```python
from build123d import *

# Parameters (mm, degrees)
BOSS_EXTRUDE1_DEPTH    = 42
SKETCH4_W              = 14.859
SKETCH4_H              = 30
CUT_EXTRUDE2_DEPTH     = 6.35
SKETCH6_R              = 2.35
CUT_EXTRUDE3_DEPTH     = 6.35
CUT_EXTRUDE4_REACH     = 49.295
SKETCH7_R              = 1.625
CONVERT_SOLID1_DEPTH   = 6.254
CONVERT_SOLID1_START   = 35.746
CONVERT_SOLID1_2_DEPTH = 6.254
CONVERT_SOLID1_START_2 = 5.746
CONVERT_SOLID1_3_DEPTH = 0.508
CONVERT_SOLID1_4_DEPTH = 0.508
CONVERT_SOLID1_5_DEPTH = 5.746
CONVERT_SOLID1_START_3 = 36.254
CONVERT_SOLID1_6_DEPTH = 5.746


# Read off the part's stored shape, not the designer's step: Convert-Solid1
with BuildPart() as part:
    # Sketch1 → Boss-Extrude1 (new body)
    with BuildSketch(Plane(origin=(0, 0, 0), x_dir=(1, 0, 0), z_dir=(0, 1, 0))):
        Polygon((0, 0), (15.875, 0), (15.875, 1.016), (1.016, 1.016), (1.016, 15.875), (0, 15.875), align=None)
    extrude(amount=BOSS_EXTRUDE1_DEPTH)

    # Sketch4 → Cut-Extrude2 (cut)
    with BuildSketch(Plane(origin=(1.016, 0, 0), x_dir=(0, 0, -1), z_dir=(1, 0, 0))):
        with Locations((8.4455, 21)):
            Rectangle(SKETCH4_W, SKETCH4_H)
    extrude(amount=-CUT_EXTRUDE2_DEPTH, mode=Mode.SUBTRACT)

    # Sketch6 → Cut-Extrude3 (cut)
    with BuildSketch(Plane(origin=(1.016, 0, 0), x_dir=(0, 0, -1), z_dir=(1, 0, 0))):
        with Locations((7.666, 3.35)):
            Circle(SKETCH6_R)
        with Locations((7.666, 38.65)):
            Circle(SKETCH6_R)
    extrude(amount=-CUT_EXTRUDE3_DEPTH, mode=Mode.SUBTRACT)

    # Sketch7 → Cut-Extrude4 (cut, up to next)
    with BuildSketch(Plane(origin=(0, 0, -1.016), x_dir=(-1, 0, 0), z_dir=(0, 0, -1)), mode=Mode.PRIVATE) as cut_extrude4_sk1:
        with Locations((-8.4455, 39)):
            Circle(SKETCH7_R)
    cut_extrude4_tool1 = extrude(cut_extrude4_sk1.sketch, amount=-CUT_EXTRUDE4_REACH, mode=Mode.PRIVATE) & part.part
    # Sketch7 → Cut-Extrude4 (cut, up to next)
    with BuildSketch(Plane(origin=(0, 0, -1.016), x_dir=(-1, 0, 0), z_dir=(0, 0, -1)), mode=Mode.PRIVATE) as cut_extrude4_sk2:
        with Locations((-8.4455, 3)):
            Circle(SKETCH7_R)
    cut_extrude4_tool2 = extrude(cut_extrude4_sk2.sketch, amount=-CUT_EXTRUDE4_REACH, mode=Mode.PRIVATE) & part.part
    add(cut_extrude4_tool1.solids().sort_by_distance((8.4455, 39, -1.016))[0], mode=Mode.SUBTRACT)
    add(cut_extrude4_tool2.solids().sort_by_distance((8.4455, 3, -1.016))[0], mode=Mode.SUBTRACT)

    # Convert-Solid1 outline → Convert-Solid1 (cut)
    with BuildSketch(Plane(origin=(0, 0, 0), x_dir=(1, 0, 0), z_dir=(0, 1, 0))):
        with BuildLine():
            Line((0, 0), (2.016, 0))
            ThreePointArc((2.016, 0), (0.590472729, 0.590472729), (0, 2.016))
            Line((0, 2.016), (0, 0))
        make_face()
    extrude(amount=CONVERT_SOLID1_DEPTH, mode=Mode.SUBTRACT)

    # Convert-Solid1 2 outline → Convert-Solid1 2 (cut)
    with BuildSketch(Plane(origin=(0, 0, 0), x_dir=(1, 0, 0), z_dir=(0, 1, 0)).offset(CONVERT_SOLID1_START)):
        with BuildLine():
            Line((0, 0), (2.016, 0))
            ThreePointArc((2.016, 0), (0.590472729, 0.590472729), (0, 2.016))
            Line((0, 2.016), (0, 0))
        make_face()
    extrude(amount=CONVERT_SOLID1_2_DEPTH, mode=Mode.SUBTRACT)

    # Convert-Solid1 3 outline → Convert-Solid1 3 (cut)
    with BuildSketch(Plane(origin=(0, 0, 0), x_dir=(1, 0, 0), z_dir=(0, 1, 0)).offset(CONVERT_SOLID1_START_2)):
        with BuildLine():
            Line((2.016, 0), (3.54, 0))
            Line((3.54, 0), (3.54, 1.016))
            Line((3.54, 1.016), (1.016, 1.016))
            Line((1.016, 1.016), (1.016, 3.54))
            Line((1.016, 3.54), (0, 3.54))
            Line((0, 3.54), (0, 2.016))
            ThreePointArc((0, 2.016), (0.590472729, 0.590472729), (2.016, 0))
        make_face()
    extrude(amount=CONVERT_SOLID1_3_DEPTH, mode=Mode.SUBTRACT)

    # Convert-Solid1 4 outline → Convert-Solid1 4 (cut)
    with BuildSketch(Plane(origin=(0, 0, 0), x_dir=(1, 0, 0), z_dir=(0, 1, 0)).offset(CONVERT_SOLID1_START)):
        with BuildLine():
            Line((2.016, 0), (3.54, 0))
            Line((3.54, 0), (3.54, 1.016))
            Line((3.54, 1.016), (1.016, 1.016))
            Line((1.016, 1.016), (1.016, 3.54))
            Line((1.016, 3.54), (0, 3.54))
            Line((0, 3.54), (0, 2.016))
            ThreePointArc((0, 2.016), (0.590472729, 0.590472729), (2.016, 0))
        make_face()
    extrude(amount=CONVERT_SOLID1_4_DEPTH, mode=Mode.SUBTRACT)

    # Convert-Solid1 5 outline → Convert-Solid1 5 (add)
    with BuildSketch(Plane(origin=(0, 0, 0), x_dir=(1, 0, 0), z_dir=(0, 1, 0))):
        with BuildLine():
            Line((1.016, 1.016), (2.016, 1.016))
            ThreePointArc((2.016, 1.016), (1.308893219, 1.308893219), (1.016, 2.016))
            Line((1.016, 2.016), (1.016, 1.016))
        make_face()
    extrude(amount=CONVERT_SOLID1_5_DEPTH)

    # Convert-Solid1 6 outline → Convert-Solid1 6 (add)
    with BuildSketch(Plane(origin=(0, 0, 0), x_dir=(1, 0, 0), z_dir=(0, 1, 0)).offset(CONVERT_SOLID1_START_3)):
        with BuildLine():
            Line((1.016, 1.016), (2.016, 1.016))
            ThreePointArc((2.016, 1.016), (1.308893219, 1.308893219), (1.016, 2.016))
            Line((1.016, 2.016), (1.016, 1.016))
        make_face()
    extrude(amount=CONVERT_SOLID1_6_DEPTH)


solid = part.part
```
Check sheet for the modelled part. Datum: model origin and axes. Units: mm. A direction names the side the tool comes from. Coordinates: 2 decimals unless noted, no trailing zeros. Write each loop counter-clockwise with the first axis right and the second up, starting at its lowest first coordinate (ties: lowest second). Pieces come first, ordered by that corner, then holes. Notation, with made-up numbers: (35, 85) -> (73, 85) arc R15 ccw to (73, 106) -> close; hole circle Ø11 at (-3, 52). An arc over 180 degrees is marked (long way). Use a Markdown table: item, result.
1. Tool access check on faces 1 (the flat face through (0.5, 36, -9.6)), 2 (the flat face through (1, 36.254, -1)), 3 (the flat face through (1.016, 39, -10.4)), 4 (the cylindrical face through (0.61, 39.09, -0.57)). Record the directions out of +Z, -Z, +X, -X, +Y, -Y that give a thin tool (end or side, any length) a straight path to the whole face; none if there is none.
Reported:
| item | result |
|---|---|
| face 1 | +Z, -Z, +X, -X |
| face 2 | +Z, -X |
| face 3 | -Z, +X, +Y, -Y |
| face 4 | +Z, -X, +Y |
2. Sectioned sample at B-B (z = -12.5). Enter the section's corners in (x, y).
Reported:
| item | result |
|---|---|
| outline | (0, 0) -> (1.02, 0) -> (1.02, 6) -> (0, 6) -> close; (0, 36) -> (1.02, 36) -> (1.02, 42) -> (0, 42) -> close |
3. Sectioned sample at D-D (y = 25). Enter the section's corners in (x, z) (3 decimals).
Reported:
| item | result |
|---|---|
| outline | (0, -1.016) -> (15.875, -1.016) -> (15.875, 0) -> (0, 0) -> close |
4. Sectioned sample at C-C (z = -8.25). Enter the section's corners in (x, y).
Reported:
| item | result |
|---|---|
| outline | (0, 0) -> (1.02, 0) -> (1.02, 1.07) -> (0, 1.07) -> close; (0, 5.63) -> (1.02, 5.63) -> (1.02, 6) -> (0, 6) -> close; (0, 36) -> (1.02, 36) -> (1.02, 36.37) -> (0, 36.37) -> close; (0, 40.93) -> (1.02, 40.93) -> (1.02, 42) -> (0, 42) -> close |
5. Release check for a two-part mould opening along Y. For faces 5 (the cylindrical face through (0.61, 2.83, -0.57)), 6 (the flat face through (0.8, 42, -4.4)), 7 (the flat face through (0.5, 6, -9.6)) record: pulls with the +Y half, pulls with the -Y half, needs draft (parallel to the pull), parting line crosses it, or undercut.
Reported:
| item | result |
|---|---|
| face 5 | needs draft |
| face 6 | pulls with the +Y half |
| face 7 | undercut |
6. Go/stop test with flat-tipped pins: pin 1 Ø1 at (x, y) = (7.5, 21.5) entering from +Z; pin 2 Ø3 at (x, y) = (8.45, 3) entering from +Z; pin 3 Ø6.5 at (y, z) = (40.5, -10.5) entering from +X. Record where each tip stops, or that it passes through.
Reported:
| item | result |
|---|---|
| pin 1 | stops at z = 0 |
| pin 2 | passes through |
| pin 3 | stops at x = 1.02 |
7. Scan lines: line 1 along Z through (x, y) = (14, 29.5); line 2 along X through (y, z) = (37, -14.25). Record each from-to range of solid material in increasing order.
Reported:
| item | result |
|---|---|
| line 1 | z = -1.02 to 0 |
| line 2 | x = 0 to 1.02 |
8. Sectioned sample at A-A (x = 3). Enter the section's corners in (y, z), plus the area to 3 significant figures.
Reported:
| item | result |
|---|---|
| outline | (0, -1.02) -> (5.75, -1.02) -> (5.75, 0) -> (0, 0) -> close; (6.25, -1.02) -> (35.75, -1.02) -> (35.75, 0) -> (6.25, 0) -> close; (36.25, -1.02) -> (42, -1.02) -> (42, 0) -> (36.25, 0) -> close |
| area | 41.6 mm2 |
